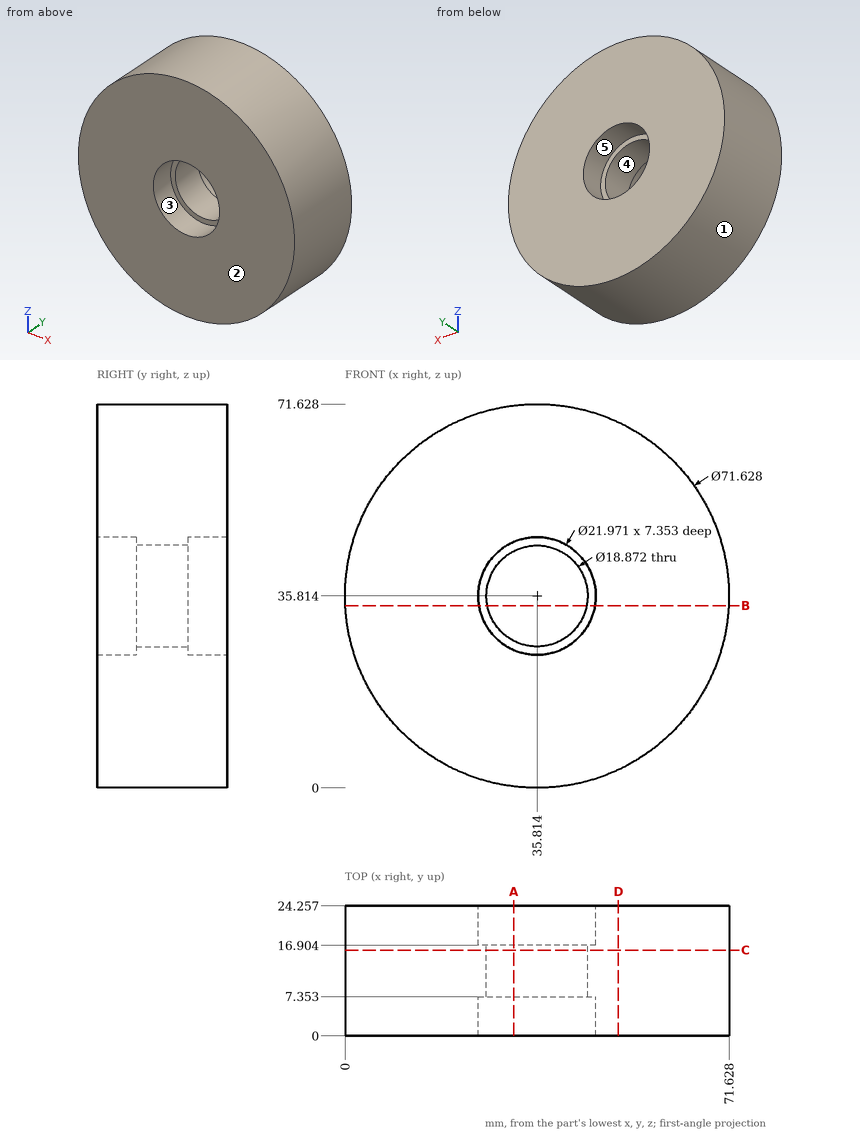
Here's the drawing with two shaded views (mm, measured from the low corner). I have some questions. A direction names the side the tool comes from. Give positions to 0.01 mm unless a question says otherwise; leave off trailing zeros. Write each loop counter-clockwise with the first axis right and the second up, starting at its lowest first coordinate (ties: lowest second). Pieces come first, ordered by that corner, then holes. Notation, with made-up numbers: (76, -7) -> (121, -7) arc R12 cw to (121, 5) -> close; hole circle Ø7 at (38, 86.5). An arc over 180 degrees is marked (long way). Answer as a JSON object with one key per item and string values. Group by question number.
Item 1: We'd pull the mould along X, two halves only. Please class the marked faces 1, 2 and 3: +X half, -X half, draft (parallel to the pull), parting line (faces both ways), or undercut.
Item 2: For the marked faces 4 and 5, which set-ups out of +Z, -Z, +X, -X, +Y, -Y let a thin tool reach every point of the face, with its end or its side?
Item 3: Suppose I cut it at B-B (z = 34). Please give me the cut outline in (x, y), plus the area to 3 significant figures.
Item 4: Please list where these lines run through material, in increasing order: line 1 (X direction, y = 19.75, z = 45); line 2 (X direction, y = 5.25, z = 37.5); line 3 (Z direction, x = 31.5, y = 17.75). Write a range as [from, to].
Item 5: Suppose I cut it at C-C (y = 16). Please give me the cut outline in (x, z).
Item 6: Suppose I cut it at D-D (x = 51). Please give me the cut outline in (y, z).
Item 7: I'm going to push flat-ended pins straight in: P1, Ø5, axis at y = 5, z = 15, coming from the +X side; P2, Ø10, axis at y = 20.5, z = 26.5, coming from the +X side; P3, Ø6, axis at y = 19, z = 46, coming from the +X side. Where does each tip first touch, or does it pass through?
Item 8: Suppose I cut it at A-A (x = 31.5). Please give me the cut outline in (y, z).
Findings:
{
 "1": {"face 1": "parting line", "face 2": "draft", "face 3": "undercut"},
 "2": {"face 4": "+Y, -Y", "face 5": "+Y"},
 "3": {"outline": "(0.05, 0) -> (24.98, 0) -> (24.98, 7.35) -> (26.55, 7.35) -> (26.55, 16.9) -> (24.98, 16.9) -> (24.98, 24.26) -> (0.05, 24.26) -> close; (45.07, 7.35) -> (46.65, 7.35) -> (46.65, 0) -> (71.58, 0) -> (71.58, 24.26) -> (46.65, 24.26) -> (46.65, 16.9) -> (45.07, 16.9) -> close", "area": "1,240 mm²"},
 "4": {"line 1": "x = [1.2, 29.79], [41.84, 70.43]", "line 2": "x = [0.04, 24.96], [46.67, 71.59]", "line 3": "z = [0.26, 25.71], [45.92, 71.37]"},
 "5": {"outline": "circle Ø71.63 at (35.81, 35.81); hole circle Ø18.87 at (35.81, 35.81)"},
 "6": {"outline": "(0, 3.38) -> (24.26, 3.38) -> (24.26, 68.25) -> (0, 68.25) -> close"},
 "7": {"P1": "stops at x = 66.59", "P2": "stops at x = 71.37", "P3": "stops at x = 70.9"},
 "8": {"outline": "(0, 0.26) -> (24.26, 0.26) -> (24.26, 25.71) -> (16.9, 25.71) -> (16.9, 27.42) -> (7.35, 27.42) -> (7.35, 25.71) -> (0, 25.71) -> close; (0, 45.92) -> (7.35, 45.92) -> (7.35, 44.21) -> (16.9, 44.21) -> (16.9, 45.92) -> (24.26, 45.92) -> (24.26, 71.37) -> (0, 71.37) -> close"}
}
